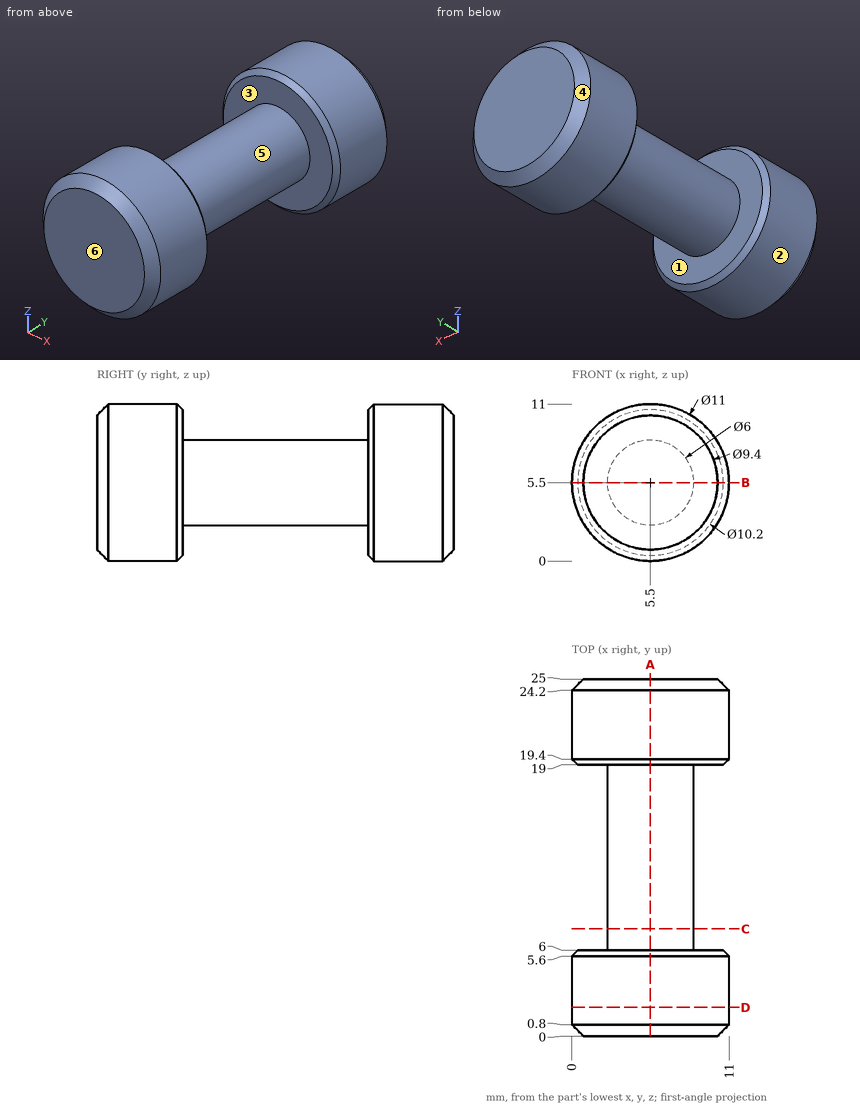
Could you check a few things on this drawing? It's one solid part, dimensions in mm from its lowest x, y, z. A direction names the side the tool comes from. Give positions to 0.01 mm unless a question says otherwise; leave off trailing zeros. Order: outer loops, then holes, each group sorted by start corner. A loop starts at its lowest first (then second) coordinate and runs counter-clockwise, first axis right, second up. Notation, with made-up numbers: (0.25, -19) - (12.25, -19) arc R16 cw to (12.25, 4) - close; hole circle Ø8 at (12, 60.25). An arc over 180 degrees is marked (long way). One line per item, written item: value. Start each with the question number.
1. Imagine slicing it at C-C on y = 7.5. List the corners of the cut face in (x, z) for me, plus the area to 3 significant figures.
2. Thinking about a two-plate mould opening in Y: for the marked faces 1, 2, 3 and 4, which applies, +Y half, -Y half, draft (parallel to the pull), parting line (faces both ways), or undercut?
3. Imagine slicing it at B-B on z = 5.5. List the corners of the cut face in (x, y) for me.
4. Imagine slicing it at A-A on x = 5.5. List the corners of the cut face in (y, z) for me.
5. Imagine slicing it at D-D on y = 2. List the corners of the cut face in (x, z) for me.
6. For P1, Ø5, axis at x = 9, y = 20.5, coming from the -Z side; P2, Ø1, axis at x = 2.5, y = 15.5, coming from the +Z side, each with a flat end and sliding along its axis, tell me the tip position at first contact or that it passes through.
7. For the marked faces 5 and 6, which set-ups out of +Z, -Z, +X, -X, +Y, -Y let a thin tool reach every point of the face, with its end or its side?
8. If I drill on probe 1 along Y at (x, z) = (8, 2); probe 2 along X at (y, z) = (10.25, 5.5); probe 3 along Y at (x, z) = (2, 1.5), over which ranges is the centre line in solid material (lowest first)?
Values:
1. outline: circle Ø6 at (5.5, 5.5)
1. area: 28.3 mm²
2. face 1: undercut
2. face 2: draft
2. face 3: undercut
2. face 4: +Y half
3. outline: (0, 0.8) - (0.8, 0) - (10.2, 0) - (11, 0.8) - (11, 5.6) - (10.6, 6) - (8.5, 6) - (8.5, 19) - (10.6, 19) - (11, 19.4) - (11, 24.2) - (10.2, 25) - (0.8, 25) - (0, 24.2) - (0, 19.4) - (0.4, 19) - (2.5, 19) - (2.5, 6) - (0.4, 6) - (0, 5.6) - close
4. outline: (0, 0.8) - (0.8, 0) - (5.6, 0) - (6, 0.4) - (6, 2.5) - (19, 2.5) - (19, 0.4) - (19.4, 0) - (24.2, 0) - (25, 0.8) - (25, 10.2) - (24.2, 11) - (19.4, 11) - (19, 10.6) - (19, 8.5) - (6, 8.5) - (6, 10.6) - (5.6, 11) - (0.8, 11) - (0, 10.2) - close
5. outline: circle Ø11 at (5.5, 5.5)
6. P1: z = 0.09
6. P2: z = 7.16
7. face 5: none
7. face 6: +Z, -Z, +X, -X, -Y
8. probe 1: 0 to 6, 19 to 25
8. probe 2: 2.5 to 8.5
8. probe 3: 0.62 to 5.78, 19.22 to 24.38
